The listing builds one solid part. Answer for the finished solid, in the listing's coordinates (mm). Face numbers are marked on the shaded views. A direction names the side the tool comes from. Round coordinates to 2 decimals unless told otherwise and drop trailing zeros. Order: outer loops, then holes, each group sorted by start corner. A loop starts at its lowest first (then second) coordinate and runs counter-clockwise, first axis right, second up. Notation, with made-up numbers: (-9.75, 55) - (11.25, 55) arc R14 ccw to (11.25, 69) - close; hole circle Ø3 at (89.25, 13). An arc over 180 degrees is marked (long way). One line per item, written item: value. Start each with the question number.
1. Straight lines are drawn through the part: line 1 (Y direction, x = -23.5, z = 9); line 2 (X direction, y = -17, z = 14); line 3 (Z direction, x = -55, y = -16.25). For each, find the intervals that lie inside material, in ascending order.
2. Section D-D, the plane x = -65 is taken. Give the vertices of the cut face in (y, z), then the cut area to 3 significant figures.
3. Section A-A, the plane z = 6 is taken. Give the vertices of the cut face in (x, y).
4. For a pull along Y with two mould halves and no side action, classify the marked faces 4, 5 and 6 as released by +Y, released by -Y, zero draft, split by the parting line, or undercut.
5. Flat-ended cylindrical pins translate along their axes: P1, Ø14, axis at x = -64, y = -14.5, coming from the +Z side; P2, Ø10, axis at x = -43.5, y = -8.5, coming from the +Z side; P3, Ø10, axis at y = -9.5, z = 22, coming from the -X side; P4, Ø1, axis at y = -14, z = 18, coming from the +X side. Find the tip coordinate at first contact, or state that the pin passes through.
6. Section B-B, the plane x = -42.5 is taken. Give the vertices of the cut face in (y, z), then the cut area to 3 significant figures.
7. Section C-C, the plane y = -17.25 is taken. Give the vertices of the cut face in (x, z).
8. A tool of negligible diameter and unlimited length cuts with its end or side. For the marked faces 1, 2 and 3, from which of +Z, -Z, +X, -X, +Y, -Y can it reach the whole face along a straight path? Write none if from no direction.
from build123d import *

# Parameters (mm, degrees)
F1_DEPTH  = 25.4
F2_R      = 6.2570868775
F3_DEPTH  = 25.4
F5_DEPTH  = 19.05
F7_DEPTH  = 19.05
F8_R      = 6.2570868775
F9_DEPTH  = 25.4
F11_DEPTH = 25.4


with BuildPart() as f1:
    # F0 (on Front) → F1 (new body)
    with BuildSketch(Plane.XZ):
        Polygon((-76.2, 0), (0, 0), (0, 12.7), (-57.15, 12.7), (-57.15, 38.1), (-76.2, 38.1), align=None)
    extrude(amount=F1_DEPTH)

    # F2 (on face) → F3 (cut)
    with BuildSketch(Plane.XY.offset(38.1)):
        with Locations((-66.675, -13.1544489413)):
            Circle(F2_R)
    extrude(amount=-F3_DEPTH, mode=Mode.SUBTRACT)

    # F4 (on face) → F5 (cut)
    with BuildSketch(Plane.XY.offset(12.7)):
        with BuildLine():
            ThreePointArc((-22.7675971567, -5.4390591716), (-29.692432865, -12.2261255428), (-22.7671458535, -19.0127314193))
            ThreePointArc((-22.7671458535, -19.0127314193), (-18.0560040915, -16.977183947), (-16.1160016177, -12.2258998454))
            ThreePointArc((-16.1160016177, -12.2258998454), (-18.0561620669, -7.4744545509), (-22.7675971567, -5.4390591716))
        make_face()
        with BuildLine():
            Line((-44.2795754893, -5.0060199297), (-44.5703677833, -5.0001662387))
            ThreePointArc((-44.5703677833, -5.0001662387), (-51.7956349782, -12.3079980641), (-44.4061819446, -19.449767865))
            ThreePointArc((-44.4061819446, -19.449767865), (-39.4032801468, -17.2768830676), (-37.3446341766, -12.2258998454))
            ThreePointArc((-37.3446341766, -12.2258998454), (-39.3592060219, -7.220400944), (-44.2795754893, -5.0060199297))
        make_face()
        with BuildLine():
            ThreePointArc((-37.3446341766, -12.2258998454), (-39.4032801468, -17.2768830676), (-44.4061819446, -19.449767865))
            Line((-44.4061819446, -19.449767865), (-22.7671458535, -19.0127314193))
            ThreePointArc((-22.7671458535, -19.0127314193), (-29.692432865, -12.2261255428), (-22.7675971567, -5.4390591716))
            Line((-22.7675971567, -5.4390591716), (-44.2795754893, -5.0060199297))
            ThreePointArc((-44.2795754893, -5.0060199297), (-39.3592060219, -7.220400944), (-37.3446341766, -12.2258998454))
        make_face()
    extrude(amount=-F5_DEPTH, mode=Mode.SUBTRACT)

    # F6 (on face) → F7 (cut)
    with BuildSketch(Plane.XY.offset(12.7)):
        with BuildLine():
            ThreePointArc((-16.7138874531, 0), (-11.8080190768, -12.761667067), (-17.0234031975, -25.4))
            Line((-17.0234031975, -25.4), (0, -25.4))
            Line((0, -25.4), (0, 0))
            Line((0, 0), (-16.7138874531, 0))
        make_face()
    extrude(amount=-F7_DEPTH, mode=Mode.SUBTRACT)

    # F8 (on face) → F9 (cut)
    with BuildSketch(Plane.XY.offset(38.1)):
        with BuildLine():
            ThreePointArc((-66.675, 0), (-57.6500295177, -12.7), (-66.675, -25.4))
            Line((-66.675, -25.4), (-57.15, -25.4))
            Line((-57.15, -25.4), (-57.15, 0))
            Line((-57.15, 0), (-66.675, 0))
        make_face()
        with BuildLine():
            Line((-76.2, -25.4), (-66.675, -25.4))
            ThreePointArc((-66.675, -25.4), (-76.0323616205, -12.7), (-66.675, 0))
            Line((-66.675, 0), (-76.2, 0))
            Line((-76.2, 0), (-76.2, -25.4))
        make_face()
        with Locations((-66.675, -13.1544489413)):
            Circle(F8_R)
    extrude(amount=-F9_DEPTH, mode=Mode.SUBTRACT)

    # F10 (on face) → F11 (cut)
    with BuildSketch(Plane.XY.offset(38.1)):
        with BuildLine():
            ThreePointArc((-73.1792891103, -4.4698874424), (-66.811491799, -1.6448572711), (-60.4505532037, -4.4852970704))
            ThreePointArc((-60.4505532037, -4.4852970704), (-63.2361374685, -1.7893568412), (-66.675, 0))
            ThreePointArc((-66.675, 0), (-70.2664103908, -1.7412661714), (-73.1792891103, -4.4698874424))
        make_face()
        with BuildLine():
            ThreePointArc((-66.675, -25.4), (-64.8290367019, -24.5975628429), (-63.1235156823, -23.5285988862))
            ThreePointArc((-63.1235156823, -23.5285988862), (-66.7799965121, -24.5102265659), (-70.439013249, -23.5380941269))
            ThreePointArc((-70.439013249, -23.5380941269), (-68.6309718215, -24.6185744834), (-66.675, -25.4))
        make_face()
    extrude(amount=-F11_DEPTH, mode=Mode.SUBTRACT)


solid = f1.part
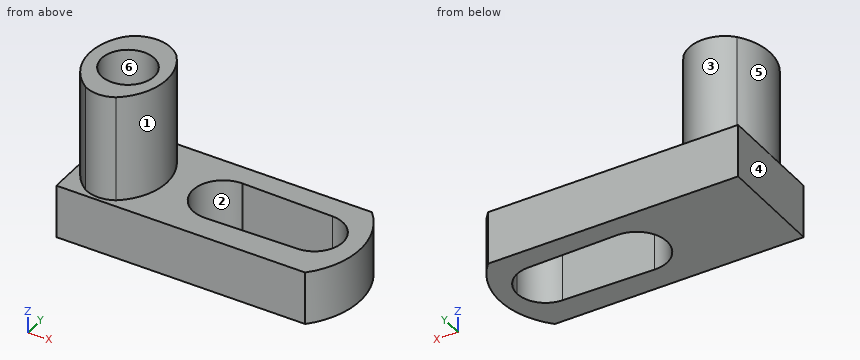
Answer list:
1. line 1: y = -25.4 to -19.03, -5.42 to 0
1. line 2: x = -75.32 to -71.61, -61.74 to -58.36
1. line 3: z = 0 to 12.7
2. outline: (-25.4, 0) - (0, 0) - (0, 12.7) - (-1.84, 12.7) - (-1.84, 38.1) - (-7.13, 38.1) - (-7.13, 12.7) - (-19.18, 12.7) - (-19.18, 38.1) - (-24.29, 38.1) - (-24.29, 12.7) - (-25.4, 12.7) - close
2. area: 586 mm²
3. outline: (-76.2, -25.4) - (-17.02, -25.4) arc R18.47 ccw to (-16.71, 0) - (-76.2, 0) - close; hole (-44.57, -5) arc R7.23 ccw (long way) to (-44.41, -19.45) - (-22.77, -19.01) arc R6.79 ccw to (-22.77, -5.44) - close
4. face 4: zero draft
4. face 5: split by the parting line
4. face 6: undercut
5. P1: stops at z = 38.1
5. P2: stops at z = 12.7
5. P3: stops at x = -76.03
5. P4: stops at x = -57.67
6. outline: (-25.4, 0) - (-19.41, 0) - (-19.41, 12.7) - (-25.4, 12.7) - close; (-5.04, 0) - (0, 0) - (0, 12.7) - (-5.04, 12.7) - close
6. area: 140 mm²
7. outline: (-76.2, 0) - (-49.76, 0) - (-49.76, 12.7) - (-58.44, 12.7) - (-58.44, 38.1) - (-61.94, 38.1) - (-61.94, 12.7) - (-71.41, 12.7) - (-71.41, 38.1) - (-75.23, 38.1) - (-75.23, 12.7) - (-76.2, 12.7) - close; (-18.34, 0) - (-12.42, 0) - (-12.42, 12.7) - (-18.34, 12.7) - close
8. face 1: +Z, +X
8. face 2: +Z, -Z
8. face 3: +Z, +Y
